For this review, take the finished solid that the model builds, in its own axes (mm). Give positions to 0.01 mm unless a question says otherwise; leave off trailing zeros. Write each loop counter-clockwise with the first axis right and the second up, starting at its lowest first coordinate (ties: lowest second). Pieces come first, ordered by that corner, then holes. Notation, with made-up numbers: M 88,-19.5 L 140,-19.5 A30 ccw 140,18.5 Z; hole C -34,25.25 d5. An arc over 180 degrees is marked long. Write item = value, one per line.
Autodesk Inventor part; units mm, degrees
ref_plane "YZ Plane" through (0, 0, 0) normal (1, 0, 0) x (0, 1, 0)
ref_plane "XZ Plane" through (0, 0, 0) normal (0, 1, 0) x (-1, 0, 0)
ref_plane "XY Plane" through (0, 0, 0) normal (0, 0, 1) x (1, 0, 0)
sketch "Sketch1" plane through (0, 0, 0) normal (0, 1, 0) x (-1, 0, 0)
  line L0 (0, 0) -> (20, 0)
  line L1 (20, 0) -> (20, 20)
  line L2 (20, 20) -> (0, 20)
  line L3 (0, 20) -> (0, 0)
  line L4 (6, 0) -> (14, 0)
  line L5 (14, 0) -> (14, 4)
  line L6 (14, 4) -> (6, 4)
  line L7 (6, 4) -> (6, 0)
  line L8 (0, 6) -> (4, 6)
  line L9 (4, 6) -> (4, 14)
  line L10 (4, 14) -> (0, 14)
  line L11 (0, 14) -> (0, 6)
  line L12 (6, 20) -> (14, 20)
  line L13 (14, 20) -> (14, 16)
  line L14 (14, 16) -> (6, 16)
  line L15 (6, 16) -> (6, 20)
  line L16 (20, 14) -> (16, 14)
  line L17 (16, 14) -> (16, 6)
  line L18 (16, 6) -> (20, 6)
  line L19 (20, 6) -> (20, 14)
  dimension "d0" = 20
  dimension "d1" = 20
  dimension "d2" = 8
  dimension "d3" = 6
  dimension "d4" = 8
  dimension "d5" = 6
  dimension "d6" = 4
  dimension "d7" = 4
  dimension "d8" = 4
  dimension "d9" = 4
extrude "Extrusion1" add sketch "Sketch1" along normal blind 381 contours L3 L8 L9 L10 L2 L15 L14 L13 L1 L16 L17 L18 L0 L5 L6 L7
fillet "Fillet1" radius 1.27 12 edges at (0, 190.5, 20) (0, 190.5, 14) (-6, 190.5, 20) (-14, 190.5, 20) (-20, 190.5, 20) (-20, 190.5, 14) (0, 190.5, 6) (0, 190.5, 0) (-6, 190.5, 0) (-14, 190.5, 0) (-20, 190.5, 0) (-20, 190.5, 6)
properties part number "20x20extrusion" material "Aluminum 6061"
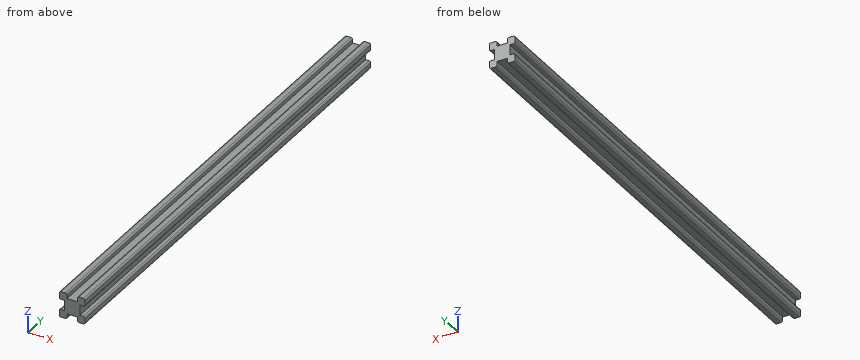
1. We need section B-B, the plane x = -10.75. Write out the cut boundary in (y, z), then the cut area to 3 significant figures.
Responses:
outline = M 0,4 L 381,4 L 381,16 L 0,16 Z
area = 4,570 mm2
2. For line 1 along X through (y, z) = (250, 17.5); line 2 along Z through (x, y) = (-2, 95.5); line 3 along X through (y, z) = (63, 13), list the stretches that pass through material, from the lowest coordinate up. Write a range as from..to.
Responses:
line_1 = -20..-14, -6..0
line_2 = 0..6, 14..20
line_3 = -16..-4
3. Insertion check: P1, Ø0.8, axis at x = -2, y = 214, coming from the -Z side; P2, Ø4, axis at x = -8.5, y = 191.5, coming from the +Z side; P3, Ø3, axis at y = 328, z = 10, coming from the +X side. Each pin has a flat end and moves straight along its axis. Give the tip position at first contact, or say it passes through.
Responses:
P1 = 0
P2 = 16
P3 = -4
